Input: part model. Units: mm. Frame: model coordinates. Give positions to 0.01 mm unless a question says otherwise; leave off trailing zeros. Loops run counter-clockwise (first coordinate to the right, second up) from the corner with the lowest first, then second, coordinate; pieces in that order, holes last. Notation, with made-up numbers: (11, 8.25) - (15, 8.25) arc R12 ccw to (15, 30.25) - close; hole circle Ø9 at (69, -8). An arc over 180 degrees is marked (long way). Answer as a JSON object with one key per item and string values.
from build123d import *

# Parameters (mm, degrees)
BOSS_EXTRUDE1_DEPTH = 10


with BuildPart() as part:
    # Sketch2 → Boss-Extrude1 (new body)
    with BuildSketch(Plane(origin=(0, 0, 0), x_dir=(1, 0, 0), z_dir=(0, 1, 0))):
        with BuildLine():
            Line((-25, 60), (25, 60))
            ThreePointArc((25, 60), (32.071067812, 57.071067812), (35, 50))
            ThreePointArc((35, 50), (26.421356237, 0), (35, -50))
            ThreePointArc((35, -50), (32.071067812, -57.071067812), (25, -60))
            Line((25, -60), (-25, -60))
            ThreePointArc((-25, -60), (-32.071067812, -57.071067812), (-35, -50))
            ThreePointArc((-35, -50), (-26.421356237, 0), (-35, 50))
            ThreePointArc((-35, 50), (-32.071067812, 57.071067812), (-25, 60))
        make_face()
    extrude(amount=BOSS_EXTRUDE1_DEPTH)


solid = part.part
Item 1: Cut plane C-C (z = -24). Return loops of the section in (x, y).
Geometry check:
{"outline": "(-28.35, 0) - (28.35, 0) - (28.35, 10) - (-28.35, 10) - close"}
Item 2: Mould query, pull axis Z, two halves, no side actions, for faces 1 (the face through (31.99, 4.93, -57.15)), 2 (the face through (0, 5, 60)), 3 (the face through (-26.423, 4.93, 0.714)). Classes: released by +Z, released by -Z, zero draft, split by the parting line, or undercut.
Geometry check:
{"face 1": "released by -Z", "face 2": "released by +Z", "face 3": "undercut"}
Item 3: Contact query for flat-ended pins moving along their axis: P1, Ø3, axis at y = 8.5, z = 25, coming from the -X side; P2, Ø3, axis at y = 5.5, z = -6, coming from the +X side; P3, Ø6, axis at y = 7, z = -15.5, coming from the -X side. Output: stop coordinate, or through.
Geometry check:
{"P1": "stops at x = -28.78", "P2": "stops at x = 26.61", "P3": "stops at x = -27.57"}
Item 4: Cut plane B-B (z = 10). Return loops of the section in (x, y), then the cut area to 3 significant figures.
Geometry check:
{"outline": "(-26.76, 0) - (26.76, 0) - (26.76, 10) - (-26.76, 10) - close", "area": "535 mm2"}
Item 5: Material intervals for line 1 (X direction, y = 4, z = 27); line 2 (X direction, y = 2.5, z = -19), sorted ascending. Write a range as [from, to].
Geometry check:
{"line 1": "x = [-28.87, 28.87]", "line 2": "x = [-27.63, 27.63]"}
Item 6: Cut plane A-A (y = 8). Return loops of the section in (x, z).
Geometry check:
{"outline": "(-35, -50) arc R10 ccw to (-25, -60) - (25, -60) arc R10 ccw to (35, -50) arc R150 cw to (35, 50) arc R10 ccw to (25, 60) - (-25, 60) arc R10 ccw to (-35, 50) arc R150 cw to start"}
